Part model, mm, in its own coordinate system. A direction names the side the tool comes from. Coordinates: 2 decimals unless noted, no trailing zeros. Order: outer loops, then holes, each group sorted by start corner. A loop starts at its lowest first (then second) coordinate and runs counter-clockwise, first axis right, second up. Notation, with made-up numbers: M -29,84.5 L 26,84.5 A20 cw 26,112.5 Z; hole C 11.5,39 d9. An arc over 180 degrees is marked long. Answer in a Markdown table with one row per item. Add a question column.
from build123d import *

# Parameters (mm, degrees)
SKETCH1_W                    = 11
SKETCH1_H                    = 26.125
CUT_EXTRUDE1_DEPTH           = 43.506639989
CUT_EXTRUDE2_DEPTH           = 43.506639989
CUT_EXTRUDE3_DEPTH           = 43.506639989
CUT_EXTRUDE4_DEPTH           = 43.506639989
CUT_EXTRUDE5_DEPTH           = 43.506639989
CUT_EXTRUDE6_DEPTH           = 43.506639989
CUT_EXTRUDE7_DEPTH           = 43.506639989
CUT_EXTRUDE8_DEPTH           = 43.506639989
CUT_EXTRUDE9_DEPTH           = 43.506639989
CUT_EXTRUDE10_DEPTH          = 43.506639989
CUT_EXTRUDE11_DEPTH          = 43.468291129
CUT_EXTRUDE12_DEPTH          = 43.468291129
CUT_EXTRUDE13_DEPTH          = 43.468291129
SKETCH15_W                   = 16.0000508
SKETCH15_H                   = 7.5
F_6_0_6_DIAMETER_HOLE1_D     = 6
F_6_0_6_DIAMETER_HOLE1_DEPTH = 22.0000508
CUT_EXTRUDE14_DEPTH          = 45.792969961
CUT_EXTRUDE14_DEPTH_BACK     = 45.792969961
SKETCH22_R                   = 2.990861642
CUT_EXTRUDE15_DEPTH          = 45.792969961
CUT_EXTRUDE15_DEPTH_BACK     = 45.792969961
SKETCH23_R                   = 1.5
SPLIT1_START                 = 6.995955282
SPLIT1_DEPTH                 = 11


# Read off the part's stored shape, not the designer's step: Split1
with BuildPart() as part:
    # Sketch1 → Revolve1 (revolve)
    with BuildSketch(Plane(origin=(0, 0, -3.755095368), x_dir=(-1, 0, 0), z_dir=(0, 0, -1)), mode=Mode.PRIVATE) as revolve1_sk:
        with Locations((-12.495955282, 15.097655255)):
            Rectangle(SKETCH1_W, SKETCH1_H)
    revolve(revolve1_sk.sketch.rotate(Axis((17.995955282, 2.035155255, -3.755095368), (-1, 0, 0)), 270), axis=Axis((17.995955282, 2.035155255, -3.755095368), (-1, 0, 0)))

    # Sketch2 → Cut-Extrude1 (cut, through all)
    with BuildSketch(Plane.ZY.offset(-6.995955282)):
        with BuildLine():
            ThreePointArc((14.332392383, 20.8861078), (13.037730936, 22.048066331), (11.668609565, 23.121286981))
            ThreePointArc((11.668609565, 23.121286981), (11.189500109, 21.585967652), (10.468111889, 20.148487096))
            ThreePointArc((10.468111889, 20.148487096), (11.04846398, 19.677350291), (11.613220242, 19.187627099))
            ThreePointArc((11.613220242, 19.187627099), (12.903594489, 20.14767169), (14.332392383, 20.8861078))
        make_face()
    extrude(amount=-CUT_EXTRUDE1_DEPTH, mode=Mode.SUBTRACT)

    # Sketch3 → Cut-Extrude2 (cut, through all)
    with BuildSketch(Plane.ZY.offset(-6.995955282)):
        with BuildLine():
            ThreePointArc((17.331036359, 17.458860187), (16.257815709, 18.827981558), (15.095857178, 20.122643005))
            ThreePointArc((15.095857178, 20.122643005), (14.357421068, 18.693845111), (13.397376477, 17.403470864))
            ThreePointArc((13.397376477, 17.403470864), (13.887099669, 16.838714603), (14.358236474, 16.258362511))
            ThreePointArc((14.358236474, 16.258362511), (15.79571703, 16.979750731), (17.331036359, 17.458860187))
        make_face()
    extrude(amount=-CUT_EXTRUDE2_DEPTH, mode=Mode.SUBTRACT)

    # Sketch4 → Cut-Extrude3 (cut, through all)
    with BuildSketch(Plane.ZY.offset(-6.995955282)):
        with BuildLine():
            ThreePointArc((19.688988892, 13.562971103), (18.869818306, 15.097655255), (17.950328137, 16.574419867))
            ThreePointArc((17.950328137, 16.574419867), (16.97500238, 15.295556708), (15.805471888, 14.191496139))
            ThreePointArc((15.805471888, 14.191496139), (16.189686188, 13.550280255), (16.552888283, 12.896932968))
            ThreePointArc((16.552888283, 12.896932968), (18.093798029, 13.3577458), (19.688988892, 13.562971103))
        make_face()
    extrude(amount=-CUT_EXTRUDE3_DEPTH, mode=Mode.SUBTRACT)

    # Sketch5 → Cut-Extrude4 (cut, through all)
    with BuildSketch(Plane.ZY.offset(-6.995955282)):
        with BuildLine():
            ThreePointArc((21.334604788, 9.316815169), (20.794374351, 10.970431499), (20.145290787, 12.584428531))
            ThreePointArc((20.145290787, 12.584428531), (18.962710163, 11.494357717), (17.619229361, 10.610157148))
            ThreePointArc((17.619229361, 10.610157148), (17.886260612, 9.91196466), (18.130492286, 9.205473805))
            ThreePointArc((18.130492286, 9.205473805), (19.728011459, 9.391709686), (21.334604788, 9.316815169))
        make_face()
    extrude(amount=-CUT_EXTRUDE4_DEPTH, mode=Mode.SUBTRACT)

    # Sketch6 → Cut-Extrude5 (cut, through all)
    with BuildSketch(Plane.ZY.offset(-6.995955282)):
        with BuildLine():
            ThreePointArc((22.217882841, 4.849409683), (21.97300718, 6.571713896), (21.614052298, 8.273902864))
            ThreePointArc((21.614052298, 8.273902864), (20.26014892, 7.405745646), (18.783538793, 6.768271063))
            ThreePointArc((18.783538793, 6.768271063), (18.925273386, 6.034316198), (19.043113783, 5.296148141))
            ThreePointArc((19.043113783, 5.296148141), (20.648702571, 5.202148388), (22.217882841, 4.849409683))
        make_face()
    extrude(amount=-CUT_EXTRUDE5_DEPTH, mode=Mode.SUBTRACT)

    # Sketch7 → Cut-Extrude6 (cut, through all)
    with BuildSketch(Plane.ZY.offset(-6.995955282)):
        with BuildLine():
            ThreePointArc((22.311985094, 0.2964945), (22.369904632, 2.035155255), (22.311985094, 3.773816009))
            ThreePointArc((22.311985094, 3.773816009), (20.827896632, 3.153950904), (19.263023231, 2.78257165))
            ThreePointArc((19.263023231, 2.78257165), (19.275154632, 2.035155255), (19.263023231, 1.287738859))
            ThreePointArc((19.263023231, 1.287738859), (20.827896632, 0.916359605), (22.311985094, 0.2964945))
        make_face()
    extrude(amount=-CUT_EXTRUDE6_DEPTH, mode=Mode.SUBTRACT)

    # Sketch8 → Cut-Extrude7 (cut, through all)
    with BuildSketch(Plane.ZY.offset(-6.995955282)):
        with BuildLine():
            ThreePointArc((21.614052298, -4.203592355), (21.97300718, -2.501403387), (22.217882841, -0.779099174))
            ThreePointArc((22.217882841, -0.779099174), (20.648702571, -1.131837878), (19.043113783, -1.225837632))
            ThreePointArc((19.043113783, -1.225837632), (18.925273386, -1.964005689), (18.783538793, -2.697960554))
            ThreePointArc((18.783538793, -2.697960554), (20.26014892, -3.335435137), (21.614052298, -4.203592355))
        make_face()
    extrude(amount=-CUT_EXTRUDE7_DEPTH, mode=Mode.SUBTRACT)

    # Sketch9 → Cut-Extrude8 (cut, through all)
    with BuildSketch(Plane.ZY.offset(-6.995955282)):
        with BuildLine():
            ThreePointArc((20.145290787, -8.514118022), (20.794374351, -6.90012099), (21.334604788, -5.24650466))
            ThreePointArc((21.334604788, -5.24650466), (19.728011459, -5.321399177), (18.130492286, -5.135163296))
            ThreePointArc((18.130492286, -5.135163296), (17.886260612, -5.841654151), (17.619229361, -6.539846639))
            ThreePointArc((17.619229361, -6.539846639), (18.962710163, -7.424047208), (20.145290787, -8.514118022))
        make_face()
    extrude(amount=-CUT_EXTRUDE8_DEPTH, mode=Mode.SUBTRACT)

    # Sketch10 → Cut-Extrude9 (cut, through all)
    with BuildSketch(Plane.ZY.offset(-6.995955282)):
        with BuildLine():
            ThreePointArc((17.950328137, -12.504109358), (18.869818306, -11.027344745), (19.688988892, -9.492660594))
            ThreePointArc((19.688988892, -9.492660594), (18.093798029, -9.287435291), (16.552888283, -8.826622459))
            ThreePointArc((16.552888283, -8.826622459), (16.189686188, -9.479969745), (15.805471888, -10.12118563))
            ThreePointArc((15.805471888, -10.12118563), (16.97500238, -11.225246199), (17.950328137, -12.504109358))
        make_face()
    extrude(amount=-CUT_EXTRUDE9_DEPTH, mode=Mode.SUBTRACT)

    # Sketch11 → Cut-Extrude10 (cut, through all)
    with BuildSketch(Plane.ZY.offset(-6.995955282)):
        with BuildLine():
            ThreePointArc((-2.016434613, 28.102235716), (-3.755095368, 28.160155255), (-5.493756122, 28.102235716))
            ThreePointArc((-5.493756122, 28.102235716), (-4.873891017, 26.618147254), (-4.502511763, 25.053273853))
            ThreePointArc((-4.502511763, 25.053273853), (-3.755095368, 25.065405255), (-3.007678972, 25.053273853))
            ThreePointArc((-3.007678972, 25.053273853), (-2.636299718, 26.618147254), (-2.016434613, 28.102235716))
        make_face()
    extrude(amount=-CUT_EXTRUDE10_DEPTH, mode=Mode.SUBTRACT)

    # Sketch12 → Cut-Extrude11 (cut, through all)
    with BuildSketch(Plane.ZY.offset(-6.995955282)):
        with BuildLine():
            ThreePointArc((2.483652242, 27.40430292), (0.781463274, 27.763257802), (-0.940840939, 28.008133463))
            ThreePointArc((-0.940840939, 28.008133463), (-0.588102235, 26.438953193), (-0.494102481, 24.833364405))
            ThreePointArc((-0.494102481, 24.833364405), (0.244065576, 24.715524008), (0.978020441, 24.573789415))
            ThreePointArc((0.978020441, 24.573789415), (1.615495024, 26.050399542), (2.483652242, 27.40430292))
        make_face()
    extrude(amount=-CUT_EXTRUDE11_DEPTH, mode=Mode.SUBTRACT)

    # Sketch13 → Cut-Extrude12 (cut, through all)
    with BuildSketch(Plane.ZY.offset(-6.995955282)):
        with BuildLine():
            ThreePointArc((6.794177909, 25.935541409), (5.180180877, 26.584624973), (3.526564547, 27.12485541))
            ThreePointArc((3.526564547, 27.12485541), (3.601459064, 25.518262081), (3.415223183, 23.920742908))
            ThreePointArc((3.415223183, 23.920742908), (4.121714038, 23.676511234), (4.819906526, 23.409479983))
            ThreePointArc((4.819906526, 23.409479983), (5.704107095, 24.752960785), (6.794177909, 25.935541409))
        make_face()
    extrude(amount=-CUT_EXTRUDE12_DEPTH, mode=Mode.SUBTRACT)

    # Sketch14 → Cut-Extrude13 (cut, through all)
    with BuildSketch(Plane.ZY.offset(-6.995955282)):
        with BuildLine():
            ThreePointArc((10.784169245, 23.740578759), (9.307404632, 24.660068928), (7.772720481, 25.479239514))
            ThreePointArc((7.772720481, 25.479239514), (7.567495178, 23.884048652), (7.106682346, 22.343138906))
            ThreePointArc((7.106682346, 22.343138906), (7.760029632, 21.97993681), (8.401245517, 21.59572251))
            ThreePointArc((8.401245517, 21.59572251), (9.505306086, 22.765253002), (10.784169245, 23.740578759))
        make_face()
    extrude(amount=-CUT_EXTRUDE13_DEPTH, mode=Mode.SUBTRACT)

    # Sketch15 → Revolve2 (revolve)
    with BuildSketch(Plane.XY.offset(-3.755095368), mode=Mode.PRIVATE) as revolve2_sk:
        with Locations((-1.004070118, 5.785155255)):
            Rectangle(SKETCH15_W, SKETCH15_H)
    revolve(revolve2_sk.sketch.rotate(Axis((-9.004095518, 2.035155255, -3.755095368), (1, 0, 0)), 270), axis=Axis((-9.004095518, 2.035155255, -3.755095368), (1, 0, 0)))

    # Ø6.0 (6) Diameter Hole1
    with Locations(Plane(origin=(17.995955282, 0, 0), x_dir=(0, 0, -1), z_dir=(1, 0, 0))):
        with Locations((3.755095368, 2.035155255)):
            Hole(F_6_0_6_DIAMETER_HOLE1_D / 2, depth=F_6_0_6_DIAMETER_HOLE1_DEPTH)

    # Sketch22 → Cut-Extrude14 (cut, two sides: drawn at the far end of the back side and taken through both)
    with BuildSketch(Plane(origin=(0, 0, 0), x_dir=(0, 0, -1), z_dir=(1, 0, 0)).offset(-CUT_EXTRUDE14_DEPTH_BACK)):
        with Locations((3.766902128, 1.977678158)):
            Circle(SKETCH22_R)
    extrude(amount=CUT_EXTRUDE14_DEPTH + CUT_EXTRUDE14_DEPTH_BACK, mode=Mode.SUBTRACT)

    # Sketch23 → Cut-Extrude15 (cut, two sides: drawn at the far end of the back side and taken through both)
    with BuildSketch(Plane.XY.offset(-CUT_EXTRUDE15_DEPTH_BACK)):
        with Locations((-2.691269596, 2.301526246)):
            Circle(SKETCH23_R)
    extrude(amount=CUT_EXTRUDE15_DEPTH + CUT_EXTRUDE15_DEPTH_BACK, mode=Mode.SUBTRACT)

    # Split1 outline → Split1 (cut)
    with BuildSketch(Plane.YZ.offset(SPLIT1_START)):
        with BuildLine():
            ThreePointArc((25.053273853, -4.502511763), (-9.479969745, -23.699876923), (-10.12118563, 15.805471888))
            ThreePointArc((-10.12118563, 15.805471888), (-11.225246199, 16.97500238), (-12.504109358, 17.950328137))
            ThreePointArc((-12.504109358, 17.950328137), (-11.027344745, -26.380009041), (28.102235716, -5.493756122))
            ThreePointArc((28.102235716, -5.493756122), (26.618147254, -4.873891017), (25.053273853, -4.502511763))
        make_face()
    extrude(amount=SPLIT1_DEPTH, mode=Mode.SUBTRACT)


solid = part.part
(1) Slice it at B-B (x = 6). List the corners of the cut face in (y, z), and give its area (3 significant figures).
(2) Slice it at D-D (z = -16). List the corners of the cut face in (x, y), and give its area (3 significant figures).
(3) Slice it at C-C (y = 6). List the corners of the cut face in (x, z), and give its area (3 significant figures).
(4) 3-axis set-ups, long thin cutter, end or side, ignore diameter. For faces 1 (the cylindrical face through (-1.885, 3.566, 1.173)), 2 (the cylindrical face through (12.419, 13.559, 16.184)), 3 (the cylindrical face through (12.42, 22.75, 9.49)), 4 (the cylindrical face through (12.419, -7.41, 18.945)): which of +Z, -Z, +X, -X, +Y, -Y reach the whole face in a straight line?
(5) Drop flat-ended pins along their axis: P1, Ø0.6, axis at y = 4, z = -4.5, coming from the +X side; P2, Ø5, axis at x = 11.5, z = 6.5, coming from the +Y side; P3, Ø5, axis at x = -2.69, y = 2.3, coming from the +Z side; P4, Ø10, axis at x = 10.5, z = 4, coming from the -Y side. Give the stop position or say it passes through.
(6) Wall check: line 1 (Y direction, x = 12.75, z = 20.5); line 2 (X direction, y = 12, z = -19.5); line 3 (Z direction, x = 12.5, y = 23). Give the ranges that are in metal, low to high.
(7) Slice it at A-A (z = -10.5). List the corners of the cut face in (x, y).
(8) Pull direction Y, two halves, no side cores. Call faces 5 (the cylindrical face through (12.419, -9.292, 18.116)), 6 (the flat face through (-9.004, -1.2, -3.9)), 7 (the cylindrical face through (12.419, 13.353, 18.072)): pulls with the +Y half, pulls with the -Y half, needs draft (parallel to the pull), parting line crosses it, or undercut.
Computed:
| question | item | result |
|---|---|---|
| 1 | outline | C 2.04,-3.76 d15; hole M 0.95,-0.96 A2.99 ccw 2.14,-6.75 A3 ccw long Z |
| 1 | area | 148 mm^2 |
| 2 | outline | M 7,-17.47 L 18,-17.47 L 18,21.54 L 7,21.54 Z |
| 2 | area | 429 mm^2 |
| 3 | outline | M -9,-10.12 L 7,-10.12 L 7,-26.44 L 18,-26.44 L 18,18.93 L 7,18.93 L 7,2.61 L -9,2.61 Z |
| 3 | area | 703 mm^2 |
| 4 | face 1 | +Z, -Z |
| 4 | face 2 | +X, -X |
| 4 | face 3 | +X, -X, +Y |
| 4 | face 4 | +Z, +X, -X |
| 5 | P1 | passes through |
| 5 | P2 | stops at y = 25.94 |
| 5 | P3 | stops at z = 3.74 |
| 5 | P4 | stops at y = -20.83 |
| 6 | line 1 | y = -5.32 to -3.47, -1.15 to 1.02, 3.05 to 5.22, 7.54 to 9.39 |
| 6 | line 2 | x = 7 to 18 |
| 6 | line 3 | z = -13.29 to 7.34, 9.78 to 11.64 |
| 7 | outline | M -9,-1.24 L 7,-1.24 L 7,-19.99 L 18,-19.99 L 18,24.06 L 7,24.06 L 7,5.31 L -9,5.31 Z; hole C -2.69,2.3 d3 |
| 8 | face 5 | pulls with the -Y half |
| 8 | face 6 | needs draft |
| 8 | face 7 | undercut |
